```python
from build123d import *

# Parameters (mm, degrees)
F1_DEPTH = 6.1
F3_DEPTH = 25


with BuildPart() as f1:
    # F0 (on Front) → F1 (new body, symmetric)
    with BuildSketch(Plane.XZ):
        with BuildLine():
            ThreePointArc((-0.013371, -1.766178), (-5.485401, -5.75), (-10.957431, -1.766178))
            Line((-10.957431, -1.766178), (-11.235401, -1.766178))
            Line((-11.235401, -1.766178), (-11.235401, -11.5))
            Line((-11.235401, -11.5), (13.251467, -11.5))
            Line((13.251467, -11.5), (13.251467, -1.766178))
            Line((13.251467, -1.766178), (13.016305, -1.766178))
            ThreePointArc((13.016305, -1.766178), (6.501467, -6.75), (-0.013371, -1.766178))
        make_face()
    extrude(amount=F1_DEPTH, both=True)

    # F2 (on face) → F3 (cut)
    with BuildSketch(Plane(origin=(0, 0, -11.5), x_dir=(1, 0, 0), z_dir=(0, 0, -1))):
        with BuildLine():
            ThreePointArc((0.64533, -0.763904), (0.907009, -0.421112), (1, 0))
            ThreePointArc((1, 0), (0.421933, 0.906627), (-0.643945, 0.765072))
            Line((-0.643945, 0.765072), (0.64533, -0.763904))
        make_face()
        with BuildLine():
            Line((0.64533, -0.763904), (-0.643945, 0.765072))
            ThreePointArc((-0.643945, 0.765072), (-0.764488, -0.644638), (0.64533, -0.763904))
        make_face()
    extrude(amount=-F3_DEPTH, mode=Mode.SUBTRACT)


solid = f1.part
```
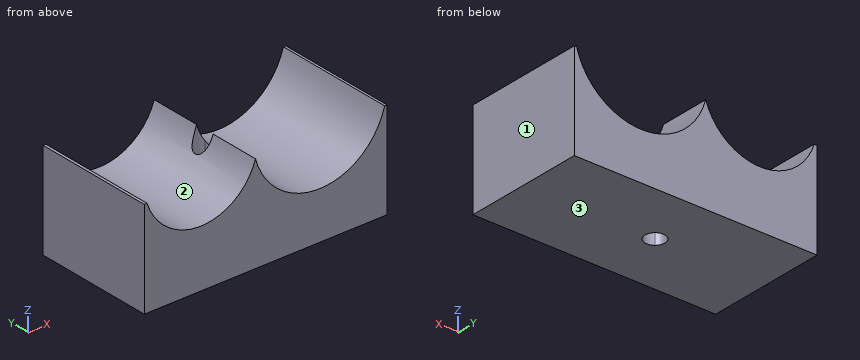
Work out the finished part from the listing and answer in its coordinate system (mm). Face numbers are marked on the shaded views. Coordinates: 2 decimals unless noted, no trailing zeros. Loops run counter-clockwise (first coordinate to the right, second up) from the corner with the lowest first, then second, coordinate; pieces in that order, holes last. Notation, with made-up numbers: M 57,79 L 105,79 A25 cw 105,91 Z; hole C -18,71 d7. An arc over 180 degrees is marked long. Use CSV: the item, a comma, the result in double quotes. Start each with the question number.
(1) Consider line 1 (X direction, y = -2.75, z = -4.5); line 2 (X direction, y = 3, z = -3.75); line 3 (Y direction, x = 0.75, z = -8.5). Determine where each line is inside the solid, lowest interval first.
(2) Find section D-D, the plane x = -2. Give the vertices of the cut face in (y, z).
(3) Find section A-A, the plane z = -5.25. Give the vertices of the cut face in (x, y), then the cut area to 3 significant figures.
(4) Given pin 1 Ø1 at (x, y) = (-7.5, -4) entering from +Z, flat-ended and moving along its own axis, determine where the tip first touches the part or whether it passes through.
(5) Find section C-C, the plane x = 3.5. Give the vertices of the cut face in (y, z).
(6) Find section B-B, the plane y = 5.25. Give the vertices of the cut face in (x, z).
(7) For a pull along X with two mould halves and no side action, classify the marked faces 1, 2 and 3 as +X half, -X half, draft (parallel to the pull), parting line (faces both ways), or undercut.
Recorded:
1,line 1,"x = -11.24 to -9.06, -1.91 to 1.47, 11.53 to 13.25"
1,line 2,"x = -11.24 to -9.84, -1.13 to 0.89, 12.11 to 13.25"
1,line 3,"y = -6.1 to -0.66, 0.66 to 6.1"
2,outline,"M -6.1,-11.5 L 6.1,-11.5 L 6.1,-4.57 L -6.1,-4.57 Z"
3,outline,"M -11.24,-6.1 L -7.83,-6.1 L -7.83,6.1 L -11.24,6.1 Z; M -3.14,-6.1 L 2.26,-6.1 L 2.26,6.1 L -3.14,6.1 Z; M 10.74,-6.1 L 13.25,-6.1 L 13.25,6.1 L 10.74,6.1 Z; hole M 0.65,0.76 A1 ccw long 1,0 A1 ccw Z"
3,area,"135 mm^2"
4,pin 1,"stops at z = -5.17"
5,outline,"M -6.1,-11.5 L 6.1,-11.5 L 6.1,-6.05 L -6.1,-6.05 Z"
6,outline,"M -11.24,-11.5 L 13.25,-11.5 L 13.25,-1.77 L 13.02,-1.77 A6.75 cw -0.01,-1.77 A5.75 cw -10.96,-1.77 L -11.24,-1.77 Z"
7,face 1,"+X half"
7,face 2,"undercut"
7,face 3,"draft"
